from build123d import *

# Parameters (mm, degrees)
F2_DEPTH     = 5.715
F3_R         = 5.08
F4_R         = 2.54
F0_R         = 3.175
F5_DEPTH     = 5.715
F7_DEPTH     = 25.4
F9_DEPTH     = 5.715
F10_T1_DEPTH = 10.4031462071
F10_T3_DEPTH = 10.4031460084
F10_T5_DEPTH = 21.8251062119
F12_DEPTH    = 12.7
F13_R        = 0.508
F15_DEPTH    = 2.54


# Not quite as in the source:
# - a fillet or chamfer that OpenCascade refuses, or shapes differently, is made with other operations: its cross-section is extruded or revolved along the edge and cut away or added


with BuildPart() as f2:
    # F1 (on Right) → F2 (new body, symmetric)
    with BuildSketch(Plane.YZ):
        Polygon((20.3924354673, 0.8880047341), (69.85, 4.8502287827), (76.2, 14.35636729), (12.8064267337, 14.35636729), (2.9200423986, 9.7313386741), (8.2383593544, 1.7451149179), (4.8682624474, -6.6303843632), (5.9557488763, -8.2313216024), align=None)
    extrude(amount=F2_DEPTH, both=True)

    # F3
    f3_edges = [f2.edges().sort_by_distance(p)[0] for p in [
        (0, 12.806427, 14.356367),
        (0, 69.85, 4.850229),
        (0, 20.392435, 0.888005),
    ]]
    fillet(f3_edges, radius=F3_R)

    # F4
    f4_edges = [f2.edges().sort_by_distance(p)[0] for p in [
        (0, 76.2, 14.356367),
    ]]
    fillet(f4_edges, radius=F4_R)

    # F0 (on Right) → F5 (join)
    with BuildSketch(Plane.YZ):
        with BuildLine():
            Line((10.16, 0), (10.033, 0))
            ThreePointArc((10.033, 0), (-1.2804712188, 9.9509538466), (-9.7061572726, -2.54))
            Line((-9.7061572726, -2.54), (-9.8373776994, -2.54))
            ThreePointArc((-9.8373776994, -2.54), (1.2802036116, -10.0790217141), (10.16, 0))
        make_face()
        Circle(F0_R, mode=Mode.SUBTRACT)
    extrude(amount=F5_DEPTH)

    # F6 (on Right) → F7 (cut)
    with BuildSketch(Plane.YZ):
        with BuildLine():
            Line((19.0573167056, 0), (5.4165862694, 8.5957078351))
            ThreePointArc((5.4165862694, 8.5957078351), (-10.1595718617, -0.0932715764), (5.5734885208, -8.4948116935))
            Line((5.5734885208, -8.4948116935), (19.0573167056, 0))
        make_face()
    extrude(amount=-F7_DEPTH, mode=Mode.SUBTRACT)

    # F8 (on Right) → F9 (join, symmetric)
    with BuildSketch(Plane.YZ):
        with BuildLine():
            Line((0.5413664183, -10.9723807834), (0.5413664183, -10.1455666378))
            ThreePointArc((0.5413664183, -10.1455666378), (-6.0054239987, -8.1951499434), (-9.8373776994, -2.54))
            Line((-9.8373776994, -2.54), (-25.4, -2.54))
            Line((-25.4, -2.54), (-25.4, -6.360667292))
            Line((-25.4, -6.360667292), (-2.5253696451, -10.9723807834))
            Line((-2.5253696451, -10.9723807834), (0.5413664183, -10.9723807834))
        make_face()
    extrude(amount=F9_DEPTH, both=True)

    # F10: fillet of radius 2.54 on 2 edges, made by hand

    # F10_s2 → F10_t1 (cut)
    with BuildSketch(Plane.YZ.offset(-10.4031461077)):
        with BuildLine():
            ThreePointArc((0.5413664183, -10.1455666378), (-0.3091706163, -10.7565034211), (-1.3338920247, -10.9723807834))
            Line((-1.3338920247, -10.9723807834), (0.5413664183, -10.9723807834))
            Line((0.5413664183, -10.9723807834), (0.5413664183, -10.1455666378))
        make_face()
    extrude(amount=F10_T1_DEPTH, mode=Mode.SUBTRACT)

    # F10_s4 → F10_t3 (cut)
    with BuildSketch(Plane.YZ.offset(9.94e-08)):
        with BuildLine():
            ThreePointArc((0.5413664183, -10.1455666378), (-0.3091706163, -10.7565034211), (-1.3338920247, -10.9723807834))
            Line((-1.3338920247, -10.9723807834), (0.5413664183, -10.9723807834))
            Line((0.5413664183, -10.9723807834), (0.5413664183, -10.1455666378))
        make_face()
    extrude(amount=F10_T3_DEPTH, mode=Mode.SUBTRACT)

    # F10_s6 → F10_t5 (cut)
    with BuildSketch(Plane.YZ.offset(-10.912553106)):
        with BuildLine():
            ThreePointArc((-23.3619846843, -6.7715479306), (-24.8255331463, -5.8904591062), (-25.4, -4.2816460496))
            Line((-25.4, -4.2816460496), (-25.4, -6.360667292))
            Line((-25.4, -6.360667292), (-23.3619846843, -6.7715479306))
        make_face()
    extrude(amount=F10_T5_DEPTH, mode=Mode.SUBTRACT)

    # F11 (on face) → F12 (join)
    with BuildSketch(Plane.XZ.offset(25.4)):
        Polygon((0, -0.4141342943), (-1.27, -2.54), (1.27, -2.54), align=None)
    extrude(amount=-F12_DEPTH)

    # F13
    f13_edges = [f2.edges().sort_by_distance(p)[0] for p in [
        (0, -19.05, -0.414134),
    ]]
    fillet(f13_edges, radius=F13_R)

    # F14 (on face) → F15 (cut)
    with BuildSketch(Plane.YZ.offset(5.715)):
        Polygon((5.715, -3.2995567884), (5.715, 3.2995567884), (0, 6.5991135768), (-5.715, 3.2995567884), (-5.715, -3.2995567884), (0, -6.5991135768), align=None)
    extrude(amount=-F15_DEPTH, mode=Mode.SUBTRACT)


solid = f2.part
The model under review builds one solid part; all positions refer to its coordinate system, in mm. A direction names the side the tool comes from. Coordinates: 2 decimals unless noted, no trailing zeros. Loops run counter-clockwise (first coordinate to the right, second up) from the corner with the lowest first, then second, coordinate; pieces in that order, holes last. Notation, with made-up numbers: (8, -20) -> (48, -20) arc R16 cw to (48, -3) -> close; hole circle Ø11 at (32.25, 19.25). An arc over 180 degrees is marked (long way). Use a Markdown table: item, result. Add a question column.
1. Add section C-C on y = 63. Write out the cut boundary in (x, z) (3 decimals), plus the area to 3 significant figures.
2. Machinability: for faces 1 (the face through (4, -5.715, 0)), 2 (the face through (0.08, 72.372, 8.626)), 3 (the face through (-2.82, 12.31, 4.25)), which of the approach directions +Z, -Z, +X, -X, +Y, -Y give a long, thin tool a straight path to every point of the face, cutting with its end or side? Answer none if there is none.
3. Add section D-D on y = 37. Write out the cut boundary in (x, z) (1 decimal).
4. Draft analysis for pull direction Z (two halves, no side actions). For faces 4 (the face through (3.175, 2, -3)), 5 (the face through (0, 4, 0)), 6 (the face through (2.62, 12.551, -4.065)), state which applies: pulls with the +Z half, pulls with the -Z half, needs draft (parallel to the pull), parting line crosses it, or undercut.
5. Add section B-B on x = -3.5. Write out the cut boundary in (y, z), plus the area to 3 significant figures.
6. To check wall thickness, follow line 1 (X direction, y = -8.5, z = 2) (3 decimals); line 2 (Z direction, x = 2.15, y = 0) (3 decimals); line 3 (Y direction, x = 1.15, z = 0) (3 decimals). State the ranges of each line that lie inside material, in increasing order.
7. Clearance check with flat-ended pins moving along their axes: pin 1 Ø0.8 at (x, z) = (4, 1.5) entering from -Y; pin 2 Ø10 at (y, z) = (3, -5.5) entering from -X; pin 3 Ø3 at (x, z) = (5, -1.5) entering from +Y. State where each tip first meets the part, or that it passes through.
Returned:
| question | item | result |
|---|---|---|
| 1 | outline | (-5.715, 4.301) -> (5.715, 4.301) -> (5.715, 14.356) -> (-5.715, 14.356) -> close |
| 1 | area | 115 mm² |
| 2 | face 1 | +X |
| 2 | face 2 | -Z, +X, -X, +Y |
| 2 | face 3 | -Z, -X, -Y |
| 3 | outline | (-5.7, 2.2) -> (5.7, 2.2) -> (5.7, 14.4) -> (-5.7, 14.4) -> close |
| 4 | face 4 | undercut |
| 4 | face 5 | needs draft |
| 4 | face 6 | pulls with the -Z half |
| 5 | outline | (-25.4, -4.28) arc R2.54 ccw to (-23.36, -6.77) -> (-2.53, -10.97) -> (-1.33, -10.97) arc R2.54 ccw to (0.54, -10.15) arc R10.16 cw to (-9.84, -2.54) -> (-25.4, -2.54) -> close; (2.92, 9.73) arc R10.16 cw to (5.42, 8.6) -> (19.02, 0.02) -> (19.33, 0.22) arc R5.08 cw to (21.64, 0.99) -> (67.4, 4.65) arc R5.08 ccw to (71.22, 6.9) -> (73.56, 10.41) arc R2.54 ccw to (71.45, 14.36) -> (13.94, 14.36) arc R5.08 ccw to (11.78, 13.88) -> close |
| 5 | area | 843 mm² |
| 6 | line 1 | x = 0 to 5.715 |
| 6 | line 2 | z = -10.594 to -3.175, 3.175 to 10.033 |
| 6 | line 3 | y = -10.033 to -3.175, 3.175 to 18.987 |
| 7 | pin 1 | stops at y = -9.97 |
| 7 | pin 2 | stops at x = 0 |
| 7 | pin 3 | stops at y = 18.99 |
